The listing builds one solid part. Answer for the finished solid, in the listing's coordinates (mm). A direction names the side the tool comes from. Round coordinates to 2 decimals unless told otherwise and drop trailing zeros. Write each loop counter-clockwise with the first axis right and the second up, starting at its lowest first coordinate (ties: lowest second). Pieces come first, ordered by that corner, then holes.
Item 1: Find the intervals of material crossed by probe 1 along Y at (x, z) = (121, 13); probe 2 along Y at (x, z) = (97.5, 92.5); probe 3 along X at (y, z) = (20, 3), in increasing order.
Item 2: Each of these flat-tipped pins is pushed along its axis until it touches: pin 1 (12 mm diameter, centred on x = 74, z = 50.5, fed in from -Y); pin 2 (2 mm diameter, centred on x = 108, z = 77.5, fed in from -Y); pin 3 (1.5 mm diameter, centred on y = -55.5, z = 65, fed in from -X); pin 4 (10 mm diameter, centred on y = 16.5, z = 82, fed in from +X). Where does it stop, or does it pass through?
Item 3: Find section B-B on y = -18. Give the vertices of the cut face in (x, z), then the cut area to 3 significant figures.
Item 4: Find section A-A on x = 86. Give the vertices of the cut face in (y, z), then the cut area to 3 significant figures.
Item 5: Find section D-D on x = 54. Give the vertices of the cut face in (y, z), then the cut area to 3 significant figures.
Item 6: For a pull along Y with two mould halves and no side action, classify faces 1 (the face through (68.703, -71.359, 48.286)), 2 (the face through (154.4, -53.3, 0)), 3 (the face through (72, 35.5, 51)) as +Y half, -Y half, draft (parallel to the pull), parting line (faces both ways), or undercut.
Item 7: A tool of negligible diameter and unlimited length cuts with its end or side. For faces 4 (the face through (72, -31.5, 51)), 5 (the face through (64, 58, 0)), 6 (the face through (125, -31.5, 49)), from which of +Z, -Z, +X, -X, +Y, -Y can it reach the whole face along a straight path? Write none if from no direction.
Item 8: Find section C-C on z = 61. Give the number of separate pieces and of enclosed holes in the cut face, then the cut area to 3 significant figures.
```python
from build123d import *

# Parameters (mm, degrees)
BOSS_EXTRU_9_DEPTH       = 100
ESQUISSE31_W             = 77
ESQUISSE31_H             = 37
ESQUISSE31_W_2           = 48
ESQUISSE31_H_2           = 67
ENL_V_MAT_EXTRU_17_DEPTH = 100
ESQUISSE35_W             = 61
ESQUISSE35_H             = 70
ENL_V_MAT_EXTRU_20_DEPTH = 2
ESQUISSE37_W             = 70
ESQUISSE37_H             = 51
ENL_V_MAT_EXTRU_22_DEPTH = 52
ESQUISSE38_W             = 61
ESQUISSE38_H             = 70
ENL_V_MAT_EXTRU_23_DEPTH = 2
ESQUISSE36_W             = 80
ESQUISSE36_H             = 21
ENL_V_MAT_EXTRU_25_DEPTH = 2
ESQUISSE39_W             = 83.5
ESQUISSE39_H             = 17
ESQUISSE39_H_2           = 19
ENL_V_MAT_EXTRU_26_DEPTH = 2
ESQUISSE46_R             = 1.5
BOSS_EXTRU_10_DEPTH      = 2
CONG_59_R                = 4


with BuildPart() as part:
    # Esquisse27 → Boss.-Extru.9 (new body)
    with BuildSketch(Plane.XY):
        Polygon((148.5, -72.5), (67.5, -72.5), (67.5, -33.5), (46.5, -33.5), (46.5, 37.5), (67.5, 37.5), (67.5, 76.5), (148.5, 76.5), (148.5, 35.5), (98.5, 35.5), (98.5, -31.5), (148.5, -31.5), align=None)
    extrude(amount=BOSS_EXTRU_9_DEPTH)

    # Esquisse31 → Enlèv. mat.-Extru.17 (cut)
    with BuildSketch(Plane.XY.offset(100)):
        with Locations((108, 56)):
            Rectangle(ESQUISSE31_W, ESQUISSE31_H)
        with Locations((72.5, 2)):
            Rectangle(ESQUISSE31_W_2, ESQUISSE31_H_2)
        with Locations((108, -52)):
            Rectangle(ESQUISSE31_W, ESQUISSE31_H)
    extrude(amount=-ENL_V_MAT_EXTRU_17_DEPTH, mode=Mode.SUBTRACT)

    # Esquisse35 → Enlèv. mat.-Extru.20 (cut)
    with BuildSketch(Plane.XZ.offset(72.5)):
        with Locations((108, 55)):
            Rectangle(ESQUISSE35_W, ESQUISSE35_H)
    extrude(amount=-ENL_V_MAT_EXTRU_20_DEPTH, mode=Mode.SUBTRACT)

    # Esquisse37 → Enlèv. mat.-Extru.22 (cut)
    with BuildSketch(Plane.ZY.offset(-46.5)):
        with Locations((55, 2)):
            Rectangle(ESQUISSE37_W, ESQUISSE37_H)
    extrude(amount=-ENL_V_MAT_EXTRU_22_DEPTH, mode=Mode.SUBTRACT)

    # Esquisse38 → Enlèv. mat.-Extru.23 (cut)
    with BuildSketch(Plane(origin=(0, 76.5, 0), x_dir=(1, 0, 0), z_dir=(0, 1, 0))):
        with Locations((108, -55)):
            Rectangle(ESQUISSE38_W, ESQUISSE38_H)
    extrude(amount=-ENL_V_MAT_EXTRU_23_DEPTH, mode=Mode.SUBTRACT)

    # Esquisse36 → Enlèv. mat.-Extru.25 (cut)
    with BuildSketch(Plane.ZY.offset(-67.5)):
        with Locations((50, 58)):
            Rectangle(ESQUISSE36_W, ESQUISSE36_H)
        with Locations((50, -54)):
            Rectangle(ESQUISSE36_W, ESQUISSE36_H)
    extrude(amount=-ENL_V_MAT_EXTRU_25_DEPTH, mode=Mode.SUBTRACT)

    # Esquisse39 → Enlèv. mat.-Extru.26 (cut)
    with BuildSketch(Plane(origin=(148.5, 0, 0), x_dir=(0, 0, -1), z_dir=(1, 0, 0))):
        with Locations((-58.25, 46)):
            Rectangle(ESQUISSE39_W, ESQUISSE39_H)
        with Locations((-58.25, -43)):
            Rectangle(ESQUISSE39_W, ESQUISSE39_H_2)
    extrude(amount=-ENL_V_MAT_EXTRU_26_DEPTH, mode=Mode.SUBTRACT)

    # Esquisse46 → Boss.-Extru.10 (add)
    with BuildSketch(Plane(origin=(0, 0, 0), x_dir=(-1, 0, 0), z_dir=(0, 0, -1))):
        with BuildLine():
            Line((-148.5, 64.356406461), (-148.5, 76.5))
            Line((-148.5, 76.5), (-114.92820323, 76.5))
            Line((-114.92820323, 76.5), (-114.92820323, 84.5))
            ThreePointArc((-114.92820323, 84.5), (-108, 88.5), (-101.07179677, 84.5))
            Line((-101.07179677, 84.5), (-101.07179677, 76.5))
            Line((-101.07179677, 76.5), (-67.5, 76.5))
            Line((-67.5, 76.5), (-67.5, 68.5))
            Line((-67.5, 68.5), (-61.5, 68.5))
            Line((-61.5, 68.5), (-61.5, 59.8))
            ThreePointArc((-61.5, 59.8), (-57.55122926, 53.5), (-61.5, 47.2))
            Line((-61.5, 47.2), (-67.5, 47.2))
            Line((-67.5, 47.2), (-67.5, 37.5))
            Line((-67.5, 37.5), (-46.5, 37.5))
            Line((-46.5, 37.5), (-46.5, -33.5))
            Line((-46.5, -33.5), (-67.5, -33.5))
            Line((-67.5, -33.5), (-67.5, -43.199792715))
            Line((-67.5, -43.199792715), (-61.5, -43.199792715))
            ThreePointArc((-61.5, -43.199792715), (-57.551027919, -49.556334189), (-61.60179677, -55.848493732))
            Line((-61.60179677, -55.848493732), (-61.60179677, -64.5))
            Line((-61.60179677, -64.5), (-67.5, -64.5))
            Line((-67.5, -64.5), (-67.5, -72.5))
            Line((-67.5, -72.5), (-100.97, -72.5))
            Line((-100.97, -72.5), (-100.97, -80.5))
            ThreePointArc((-100.97, -80.5), (-107.89820323, -84.5), (-114.826406461, -80.5))
            Line((-114.826406461, -80.5), (-114.826406461, -72.5))
            Line((-114.826406461, -72.5), (-148.5, -72.5))
            Line((-148.5, -72.5), (-148.5, -60.356406461))
            Line((-148.5, -60.356406461), (-156.5, -60.356406461))
            ThreePointArc((-156.5, -60.356406461), (-160.5, -53.42820323), (-156.5, -46.5))
            Line((-156.5, -46.5), (-148.5, -46.5))
            Line((-148.5, -46.5), (-148.5, 50.5))
            Line((-148.5, 50.5), (-156.5, 50.5))
            ThreePointArc((-156.5, 50.5), (-160.5, 57.42820323), (-156.5, 64.356406461))
            Line((-156.5, 64.356406461), (-148.5, 64.356406461))
        make_face()
        with Locations((-108, 80.5)):
            Circle(ESQUISSE46_R, mode=Mode.SUBTRACT)
        with Locations((-152.5, 57.42820323)):
            Circle(ESQUISSE46_R, mode=Mode.SUBTRACT)
        with Locations((-64.55122926, 53.5)):
            Circle(ESQUISSE46_R, mode=Mode.SUBTRACT)
        with Locations(Location((-64.550801234, -49.5, 0), (0, 0, 180))):
            Circle(ESQUISSE46_R, mode=Mode.SUBTRACT)
        with Locations(Location((-152.5, -53.42820323, 0), (0, 0, 180))):
            Circle(ESQUISSE46_R, mode=Mode.SUBTRACT)
        with Locations(Location((-107.89820323, -76.5, 0), (0, 0, 180))):
            Circle(ESQUISSE46_R, mode=Mode.SUBTRACT)
    extrude(amount=BOSS_EXTRU_10_DEPTH)

    # Congé59
    cong_59_edges = [part.edges().sort_by_distance(p)[0] for p in [
        (98.5, 35.5, 50),
        (98.5, -31.5, 50),
        (148.5, -72.5, 49),
        (67.5, -72.5, 49),
        (67.5, -33.5, 49),
        (46.5, -33.5, 49),
        (46.5, 37.5, 49),
        (67.5, 37.5, 49),
        (67.5, 76.5, 49),
        (148.5, 76.5, 49),
        (61.5, 68.5, -1),
        (61.60179677, -64.5, -1),
    ]]
    fillet(cong_59_edges, radius=CONG_59_R)


solid = part.part
```
Check values:
1. probe 1: y = -72.5 to -70.5, -33.5 to -31.5, 35.5 to 37.5, 74.5 to 76.5
1. probe 2: y = -72.5 to -70.5, -33.5 to 37.5, 74.5 to 76.5
1. probe 3: x = 46.5 to 48.5, 96.5 to 98.5
2. pin 1: stops at y = -72.5
2. pin 2: stops at y = -33.5
2. pin 3: stops at x = 146.5
2. pin 4: passes through
3. outline: (46.5, -2) - (148.5, -2) - (148.5, 0) - (98.5, 0) - (98.5, 20) - (96.5, 20) - (96.5, 0) - (48.5, 0) - (48.5, 20) - (46.5, 20) - close; (46.5, 90) - (48.5, 90) - (48.5, 100) - (46.5, 100) - close; (96.5, 90) - (98.5, 90) - (98.5, 100) - (96.5, 100) - close
3. area: 324 mm2
4. outline: (-72.5, -2) - (76.5, -2) - (76.5, 20) - (74.5, 20) - (74.5, 0) - (37.5, 0) - (37.5, 100) - (35.5, 100) - (35.5, 0) - (-31.5, 0) - (-31.5, 100) - (-33.5, 100) - (-33.5, 0) - (-70.5, 0) - (-70.5, 20) - (-72.5, 20) - close; (-72.5, 90) - (-70.5, 90) - (-70.5, 100) - (-72.5, 100) - close; (74.5, 90) - (76.5, 90) - (76.5, 100) - (74.5, 100) - close
4. area: 818 mm2
5. outline: (-33.5, -2) - (37.5, -2) - (37.5, 100) - (35.5, 100) - (35.5, 0) - (-31.5, 0) - (-31.5, 100) - (-33.5, 100) - close
5. area: 542 mm2
6. face 1: -Y half
6. face 2: draft
6. face 3: undercut
7. face 4: +Z
7. face 5: +Z, -X, +Y
7. face 6: +Z, +X
8. separate pieces: 6
8. enclosed holes: 0
8. area: 685 mm2
